Geometry check sheet. Reference: the model listing, model coordinates, mm. Face numbers are marked on the shaded views. A direction names the side the tool comes from. Round coordinates to 2 decimals unless told otherwise and drop trailing zeros. Order: outer loops, then holes, each group sorted by start corner. A loop starts at its lowest first (then second) coordinate and runs counter-clockwise, first axis right, second up.
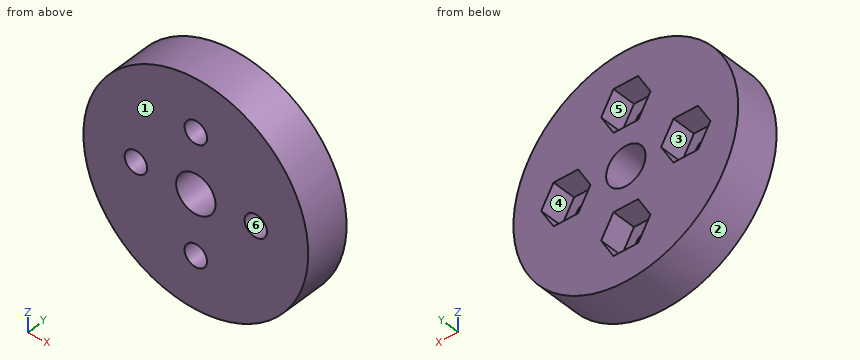
```python
from build123d import *

# Parameters (mm, degrees)
SKETCH1_R           = 15
SKETCH1_R_2         = 1.5
SKETCH1_R_3         = 2.625
BOSS_EXTRUDE1_DEPTH = 6
CUT_EXTRUDE1_DEPTH  = 3.2


with BuildPart() as part:
    # Sketch1 → Boss-Extrude1 (new body)
    with BuildSketch(Plane(origin=(0, 0, 0), x_dir=(1, 0, 0), z_dir=(0, 1, 0))):
        with Locations(Location((0, 0, 0), (0, 0, 270))):
            Circle(SKETCH1_R)
        with Locations(Location((0, 8, 0), (0, 0, 270))):
            Circle(SKETCH1_R_2, mode=Mode.SUBTRACT)
        with Locations(Location((8, 0, 0), (0, 0, 270))):
            Circle(SKETCH1_R_2, mode=Mode.SUBTRACT)
        with Locations(Location((0, -8, 0), (0, 0, 270))):
            Circle(SKETCH1_R_2, mode=Mode.SUBTRACT)
        with Locations(Location((-8, 0, 0), (0, 0, 270))):
            Circle(SKETCH1_R_2, mode=Mode.SUBTRACT)
        with Locations(Location((0, 0, 0), (0, 0, 270))):
            Circle(SKETCH1_R_3, mode=Mode.SUBTRACT)
    extrude(amount=BOSS_EXTRUDE1_DEPTH)

    # Sketch2 → Cut-Extrude1 (cut)
    with BuildSketch(Plane(origin=(0, 6, 0), x_dir=(1, 0, 0), z_dir=(0, 1, 0))):
        Polygon((3.290896534, 8), (1.645448267, 10.85), (-1.645448267, 10.85), (-3.290896534, 8), (-1.645448267, 5.15), (1.645448267, 5.15), align=None)
        Polygon((11.290896534, 0), (9.645448267, 2.85), (6.354551733, 2.85), (4.709103466, 0), (6.354551733, -2.85), (9.645448267, -2.85), align=None)
        Polygon((-4.709103466, 0), (-6.354551733, 2.85), (-9.645448267, 2.85), (-11.290896534, 0), (-9.645448267, -2.85), (-6.354551733, -2.85), align=None)
        Polygon((3.290896534, -8), (1.645448267, -5.15), (-1.645448267, -5.15), (-3.290896534, -8), (-1.645448267, -10.85), (1.645448267, -10.85), align=None)
    extrude(amount=-CUT_EXTRUDE1_DEPTH, mode=Mode.SUBTRACT)


solid = part.part
```
(1) Sectioned sample at A-A, the plane x = -2. Record the cut outline in (y, z).
Returned:
outline: (0, -14.87) - (6, -14.87) - (6, -10.24) - (2.8, -10.24) - (2.8, -5.76) - (6, -5.76) - (6, -1.7) - (0, -1.7) - close; (0, 1.7) - (6, 1.7) - (6, 5.76) - (2.8, 5.76) - (2.8, 10.24) - (6, 10.24) - (6, 14.87) - (0, 14.87) - close
(2) Sectioned sample at C-C, the plane z = -5.5. Record the cut outline in (x, y).
Returned:
outline: (-13.96, 0) - (13.96, 0) - (13.96, 6) - (1.85, 6) - (1.85, 2.8) - (-1.85, 2.8) - (-1.85, 6) - (-13.96, 6) - close
(3) Material ranges on line 1 (X direction, y = 1.95, z = 0) (3 decimals); line 2 (Z direction, x = -1.25, y = 4.3); line 3 (Z direction, x = 8.25, y = 3.65), recorded low to high.
Returned:
line 1: x = -15 to -9.5, -6.5 to -2.625, 2.625 to 6.5, 9.5 to 15
line 2: z = -14.95 to -10.85, -5.15 to -2.31, 2.31 to 5.15, 10.85 to 14.95
line 3: z = -12.53 to -2.85, 2.85 to 12.53
(4) Sectioned sample at B-B, the plane y = 3.95. Record the cut outline in (x, z) (3 decimals), and give its area (3 significant figures).
Returned:
outline: circle Ø30 at (0, 0); hole (-11.291, 0) - (-9.645, -2.85) - (-6.355, -2.85) - (-4.709, 0) - (-6.355, 2.85) - (-9.645, 2.85) - close; hole (-3.291, -8) - (-1.645, -10.85) - (1.645, -10.85) - (3.291, -8) - (1.645, -5.15) - (-1.645, -5.15) - close; hole (-3.291, 8) - (-1.645, 5.15) - (1.645, 5.15) - (3.291, 8) - (1.645, 10.85) - (-1.645, 10.85) - close; hole circle Ø5.25 at (0, 0); hole (4.709, 0) - (6.355, -2.85) - (9.645, -2.85) - (11.291, 0) - (9.645, 2.85) - (6.355, 2.85) - close
area: 573 mm2
(5) Depth check by flat-ended pin: P1, Ø3, axis at x = -8, z = 0.5, coming from the +Y side; P2, Ø1.5, axis at x = -2.5, z = 8, coming from the -Y side; P3, Ø2.5, axis at x = 8, y = 4.5, coming from the +Z side; P4, Ø1, axis at x = -3, y = 4, coming from the +Z side. Enter the tip coordinate at first touch or a pass-through.
Returned:
P1: stops at y = 2.8
P2: stops at y = 0
P3: stops at z = 13.4
P4: stops at z = 14.79
(6) Sectioned sample at D-D, the plane x = 8.5. Record the cut outline in (y, z), and give its area (3 significant figures).
Returned:
outline: (0, -12.36) - (6, -12.36) - (6, -2.85) - (2.8, -2.85) - (2.8, -1.41) - (0, -1.41) - close; (0, 1.41) - (2.8, 1.41) - (2.8, 2.85) - (6, 2.85) - (6, 12.36) - (0, 12.36) - close
area: 122 mm2
(7) Draft check along X on the marked faces 1, 2, 3 and 4. Enter one of: released by +X, released by -X, zero draft, split by the parting line, or undercut.
Returned:
face 1: zero draft
face 2: split by the parting line
face 3: undercut
face 4: undercut
(8) Set-up check for the marked faces 5 and 6: record each of +Z, -Z, +X, -X, +Y, -Y from which the full face is reachable in a straight line by a thin tool's end or side.
Returned:
face 5: +Y
face 6: +Y, -Y
